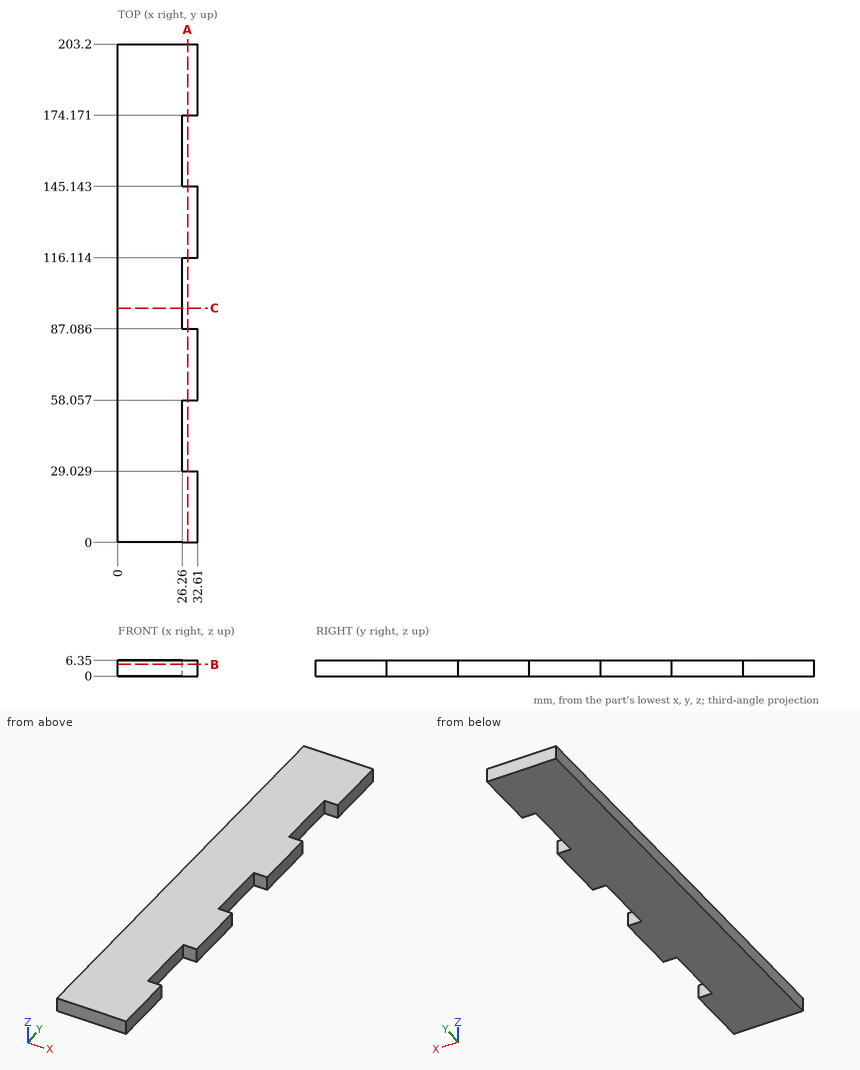
The drawing under review shows one solid part. Ordinate dimensions are in mm from its lowest x, y, z. Coordinates: 2 decimals unless noted, no trailing zeros. Write each loop counter-clockwise with the first axis right and the second up, starting at its lowest first coordinate (ties: lowest second). Pieces come first, ordered by that corner, then holes. Notation, with made-up numbers: (-15.75, 5.25) - (23.25, 5.25) arc R28 cw to (23.25, 23.25) - close; hole circle Ø4 at (76, 43). An arc over 180 degrees is marked (long way). Put each result on its own line as item: value.
1. Add section B-B, the plane z = 4.75. Give the boundary of the cut face in (x, y) (1 decimal).
Values found:
outline: (0, 0) - (32.6, 0) - (32.6, 29) - (26.3, 29) - (26.3, 58.1) - (32.6, 58.1) - (32.6, 87.1) - (26.3, 87.1) - (26.3, 116.1) - (32.6, 116.1) - (32.6, 145.1) - (26.3, 145.1) - (26.3, 174.2) - (32.6, 174.2) - (32.6, 203.2) - (0, 203.2) - close
2. Wall thickness on probe 1 along Y at (x, z) = (26.5, 5.5) (1 decimal); probe 2 along X at (y, z) = (173, 5): over which ranges is each line inside the solid? List them lowest first.
Values found:
probe 1: 0 to 29, 58.1 to 87.1, 116.1 to 145.1, 174.2 to 203.2
probe 2: 0 to 26.26
3. Add section C-C, the plane y = 95.5. Give the boundary of the cut face in (x, z).
Values found:
outline: (0, 0) - (26.26, 0) - (26.26, 6.35) - (0, 6.35) - close
4. For pin 1 (2 mm diameter, centred on x = 29, y = 102, fed in from +Z), flat-tipped, find the tip position at first contact; note if it passes through.
Values found:
pin 1: through
5. Add section A-A, the plane x = 28.5. Count the separate pieces of the cut face and the enclosed holes in it.
Values found:
separate pieces: 4
enclosed holes: 0
